Source: CAD feature listing. Evaluate the final solid. Frame: model axes, mm. Face numbers are marked on the shaded views. A direction names the side the tool comes from. Give positions to 0.01 mm unless a question says otherwise; leave off trailing zeros. Write each loop counter-clockwise with the first axis right and the second up, starting at its lowest first coordinate (ties: lowest second). Pieces come first, ordered by that corner, then holes. Notation, with made-up numbers: (46, 80.5) -> (89, 80.5) arc R18 ccw to (89, 106.5) -> close; hole circle Ø9 at (36, 24). An arc over 180 degrees is marked (long way). Write item = value, one per line.
from build123d import *

# Parameters (mm, degrees)
BOSS_EXTRUDE1_DEPTH = 50
BOSS_EXTRUDE2_START = -35
BOSS_EXTRUDE2_DEPTH = 35.000012
CUT_EXTRUDE1_DEPTH  = 15
CUT_EXTRUDE2_DEPTH  = 15
SKETCH6_R           = 20
BOSS_EXTRUDE3_DEPTH = 50
CUT_EXTRUDE4_DEPTH  = 30
BOSS_EXTRUDE4_DEPTH = 30


with BuildPart() as part:
    # Sketch1 → Boss-Extrude1 (new body)
    with BuildSketch(Plane.XY):
        Polygon((0, 0), (11, 0), (11, 32), (69, 32), (69, 0), (80, 0), (80, 55), (0, 55), align=None)
    extrude(amount=-BOSS_EXTRUDE1_DEPTH)

    # Sketch2 → Boss-Extrude2 (add)
    with BuildSketch(Plane.XY.offset(BOSS_EXTRUDE2_START)):
        Polygon((0, 0), (-20, 0), (-20, 20), (-10.43, 65), (2.57, 65), (2.57, 55), (0, 55), align=None)
        Polygon((80, 0), (100, 0), (100, 20), (90.43, 65), (77.43, 65), (77.43, 55), (80, 55), align=None)
    extrude(amount=BOSS_EXTRUDE2_DEPTH)

    # Sketch3 → Cut-Extrude1 (cut)
    with BuildSketch(Plane.XY.offset(1.2e-05)):
        Polygon((0, 0), (0, 55), (2.57, 55), (2.57, 65), (-10.43, 65), (-20, 20), (-20, 0), align=None)
    extrude(amount=-CUT_EXTRUDE1_DEPTH, mode=Mode.SUBTRACT)

    # Sketch4 → Cut-Extrude2 (cut)
    with BuildSketch(Plane.XY):
        Polygon((80, 55), (80, 0), (100, 0), (100, 20), (90.43, 65), (77.43, 65), (77.43, 55), align=None)
    extrude(amount=-CUT_EXTRUDE2_DEPTH, mode=Mode.SUBTRACT)


with BuildPart() as cut_extrude2_kept_piece:
    # of the separate pieces the step leaves, the one the design keeps (cut_extrude2_pieces_kept)
    add(part.part.solids().sort_by_distance((0, 0, -35))[0])

    # Sketch6 → Boss-Extrude3 (add)
    with BuildSketch(Plane.XY):
        with Locations((40, 55)):
            Circle(SKETCH6_R)
    extrude(amount=-BOSS_EXTRUDE3_DEPTH)

    # Sketch8 → Cut-Extrude4 (cut)
    with BuildSketch(Plane.XY):
        with BuildLine():
            Line((20, 55), (60, 55))
            ThreePointArc((60, 55), (40, 75), (20, 55))
        make_face()
    extrude(amount=-CUT_EXTRUDE4_DEPTH, mode=Mode.SUBTRACT)

    # Sketch9 → Boss-Extrude4 (add)
    with BuildSketch(Plane.XY):
        with BuildLine():
            Line((20, 55), (33.6, 55))
            Line((33.6, 55), (33.6, 65))
            Line((33.6, 65), (22.679491924, 65))
            ThreePointArc((22.679491924, 65), (20.681483474, 60.176380902), (20, 55))
        make_face()
        with BuildLine():
            Line((60, 55), (46.4, 55))
            Line((46.4, 55), (46.4, 65))
            Line((46.4, 65), (57.320508076, 65))
            ThreePointArc((57.320508076, 65), (59.318516526, 60.176380902), (60, 55))
        make_face()
    extrude(amount=-BOSS_EXTRUDE4_DEPTH)


solid = cut_extrude2_kept_piece.part
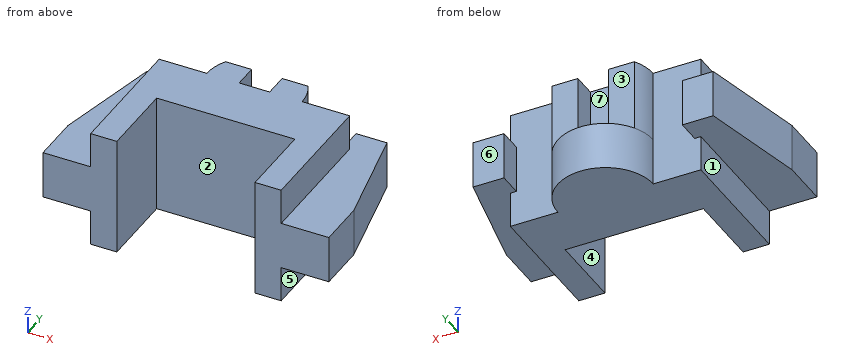
(1) Access query for the marked faces 4, 5, 6 and 7. Directions: +Z, -Z, +X, -X, +Y, -Y. A direction counts if a zero-diameter tool reaches every point of the face in a straight line with its end or side. Return the directions, or none.
Values follow:
face_4 = +Z, -Z, -Y
face_5 = -Z, +X, +Y, -Y
face_6 = +Z, -Z, +X, +Y
face_7 = +Z, +Y
(2) Section query A-A (y = 30). Return loops of the section in (x, z), plus the area to 3 significant figures.
Values follow:
outline = (-17.87, -35) -> (0, -35) -> (0, -50) -> (11, -50) -> (11, 0) -> (0, 0) -> (0, -15) -> (-17.87, -15) -> close; (69, -50) -> (80, -50) -> (80, -35) -> (97.87, -35) -> (97.87, -15) -> (80, -15) -> (80, 0) -> (69, 0) -> close
area = 1,810 mm2
(3) Section query D-D (z = -8). Return loops of the section in (x, y), plus the area to 3 significant figures.
Values follow:
outline = (0, 0) -> (11, 0) -> (11, 32) -> (69, 32) -> (69, 0) -> (80, 0) -> (80, 55) -> (60, 55) arc R20 ccw to (57.32, 65) -> (46.4, 65) -> (46.4, 55) -> (33.6, 55) -> (33.6, 65) -> (22.68, 65) arc R20 ccw to (20, 55) -> (0, 55) -> close
area = 2,800 mm2
(4) Material intervals for line 1 (X direction, y = 16.5, z = -6); line 2 (X direction, y = 20, z = -18.5); line 3 (X direction, y = 58, z = -30.5), sorted ascending.
Values follow:
line_1 = 0 to 11, 69 to 80
line_2 = -20 to 11, 69 to 100
line_3 = -11.92 to 2.57, 20.23 to 59.77, 77.43 to 91.92
(5) Section query C-C (x = 40). Return loops of the section in (y, z).
Values follow:
outline = (32, -50) -> (75, -50) -> (75, -30) -> (55, -30) -> (55, 0) -> (32, 0) -> close
(6) Section query B-B (z = -41.5). Return loops of the section in (x, y), plus the area to 3 significant figures.
Values follow:
outline = (0, 0) -> (11, 0) -> (11, 32) -> (69, 32) -> (69, 0) -> (80, 0) -> (80, 55) -> (60, 55) arc R20 ccw to (20, 55) -> (0, 55) -> close
area = 3,170 mm2
(7) First-contact query: pin 1 (8 mm diameter, centred on y = 60.5, z = -10.5, fed in from +X); pin 2 (10.5 mm diameter, centred on x = -3.5, z = -29, fed in from +Y); pin 3 (8 mm diameter, centred on y = 60.5, z = -18, fed in from -X). Flat tips, straight axial feed; report the tip coordinate or a pass-through.
Values follow:
pin_1 = 59.94
pin_2 = 65
pin_3 = -12.24
(8) Pull-direction query (X, two-part tool) for the marked faces 1, 2 and 3; classes: pulls with the +X half, pulls with the -X half, needs draft (parallel to the pull), parting line crosses it, or undercut.
Values follow:
face_1 = pulls with the -X half
face_2 = undercut
face_3 = needs draft
